Verification items for the finished model (mm, model axes). Face numbers are marked on the shaded views. A direction names the side the tool comes from. Coordinates: 2 decimals unless noted, no trailing zeros. Write each loop counter-clockwise with the first axis right and the second up, starting at its lowest first coordinate (ties: lowest second). Pieces come first, ordered by that corner, then holes. Notation, with made-up numbers: (-38, 47) -> (1, 47) arc R32 ccw to (1, 86) -> close; hole circle Ø3 at (-29.75, 52). An arc over 180 degrees is marked (long way). Answer in a Markdown table with one row per item.
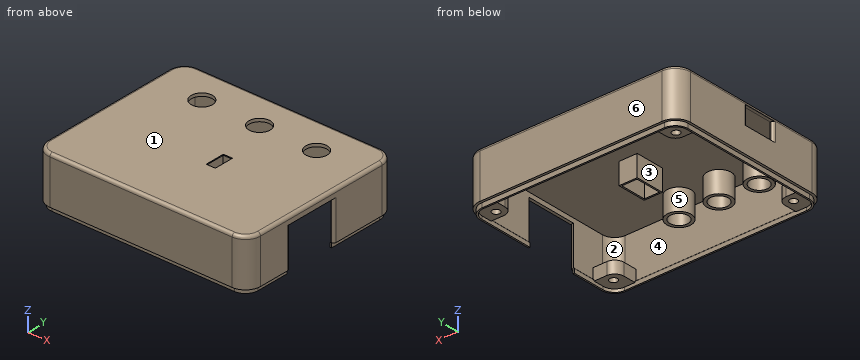
```python
from build123d import *

# Parameters (mm, degrees)
CYLINDER019_R     = 1.25
CYLINDER019_DEPTH = 10
CYLINDER018_R     = 1.25
CYLINDER018_DEPTH = 10
CYLINDER017_R     = 1.25
CYLINDER017_DEPTH = 10
BOX005_W          = 5
BOX005_H          = 8.5
BOX005_DEPTH      = 13.5
BOX006_W          = 3
BOX006_H          = 6.5
BOX006_DEPTH      = 14.5
CYLINDER015_R     = 3
CYLINDER015_DEPTH = 7.6
CYLINDER013_R     = 3
CYLINDER013_DEPTH = 7.6
CYLINDER011_R     = 3
CYLINDER011_DEPTH = 7.6
BOX003_W          = 10
BOX003_H          = 10
BOX003_DEPTH      = 6
CYLINDER002_R     = 3.5
CYLINDER002_DEPTH = 10
CYLINDER001_R     = 3.5
CYLINDER001_DEPTH = 10
CYLINDER_R        = 3.5
CYLINDER_DEPTH    = 10
BOX001_W          = 24
BOX001_H          = 16.8
BOX001_DEPTH      = 14.5
CYLINDER020_R     = 1.25
CYLINDER020_DEPTH = 10
BOX011_W          = 7.5
BOX011_H          = 7.5
BOX011_DEPTH      = 4
FILLET003_1_R     = 4
FILLET003_2_R     = 3
BOX010_W          = 7.5
BOX010_H          = 7.5
BOX010_DEPTH      = 4
FILLET002_1_R     = 4
FILLET002_2_R     = 3
BOX009_W          = 7.5
BOX009_H          = 7.5
BOX009_DEPTH      = 4
FILLET001_1_R     = 4
FILLET001_2_R     = 3
BOX004_W          = 6
BOX004_H          = 9.5
BOX004_DEPTH      = 7
CYLINDER012_R     = 4
CYLINDER012_DEPTH = 7
CYLINDER014_R     = 4
CYLINDER014_DEPTH = 7
CYLINDER016_R     = 4
CYLINDER016_DEPTH = 7
BOX008_W          = 7.5
BOX008_H          = 7.5
BOX008_DEPTH      = 4
FILLET_1_R        = 4
FILLET_2_R        = 3
BOX016_W          = 67.4
BOX016_H          = 53.4
BOX016_DEPTH      = 1.5
FILLET009_R       = 3.8
BOX013_W          = 68.4
BOX013_H          = 54.4
BOX013_DEPTH      = 1.5
FILLET008_R       = 4.2
BOX002_W          = 68
BOX002_H          = 54
BOX002_DEPTH      = 14.5
FILLET007_R       = 4
THICKNESS001_T    = 1
FILLET010_1_R     = 0.8
FILLET010_2_R     = 0.2


with BuildPart() as obj1:
    # Cylinder019 → Cylinder019 (new body)
    with BuildSketch(Plane(origin=(63.75, 49.15, -2), x_dir=(1, 0, 0), z_dir=(0, 0, 1))):
        Circle(CYLINDER019_R)
    extrude(amount=CYLINDER019_DEPTH)


with BuildPart() as obj2:
    # Cylinder018 → Cylinder018 (new body)
    with BuildSketch(Plane(origin=(4.5, 49.15, -2), x_dir=(1, 0, 0), z_dir=(0, 0, 1))):
        Circle(CYLINDER018_R)
    extrude(amount=CYLINDER018_DEPTH)


with BuildPart() as obj3:
    # Cylinder017 → Cylinder017 (new body)
    with BuildSketch(Plane(origin=(4.5, 4.65, -2), x_dir=(1, 0, 0), z_dir=(0, 0, 1))):
        Circle(CYLINDER017_R)
    extrude(amount=CYLINDER017_DEPTH)


with BuildPart() as obj4:
    # Box005 → Box005 (new body)
    with BuildSketch(Plane(origin=(35.75, 19.5, 6.2), x_dir=(1, 0, 0), z_dir=(0, 0, 1))):
        with Locations((2.5, 4.25)):
            Rectangle(BOX005_W, BOX005_H)
    extrude(amount=BOX005_DEPTH)


with BuildPart() as obj5:
    # Box006 → Box006 (new body)
    with BuildSketch(Plane(origin=(36.75, 20.5, 6.2), x_dir=(1, 0, 0), z_dir=(0, 0, 1))):
        with Locations((1.5, 3.25)):
            Rectangle(BOX006_W, BOX006_H)
    extrude(amount=BOX006_DEPTH)

    # Fusion: union obj4
    add(obj4.part)


with BuildPart() as ledhole002:
    # Cylinder015 → Cylinder015 (new body)
    with BuildSketch(Plane(origin=(40.9, 6.2, 12), x_dir=(1, 0, 0), z_dir=(0, 0, 1))):
        Circle(CYLINDER015_R)
    extrude(amount=CYLINDER015_DEPTH)


with BuildPart() as ledhole001:
    # Cylinder013 → Cylinder013 (new body)
    with BuildSketch(Plane(origin=(27.7, 6.2, 12), x_dir=(1, 0, 0), z_dir=(0, 0, 1))):
        Circle(CYLINDER013_R)
    extrude(amount=CYLINDER013_DEPTH)


with BuildPart() as ledhole:
    # Cylinder011 → Cylinder011 (new body)
    with BuildSketch(Plane(origin=(14.5, 6.2, 12), x_dir=(1, 0, 0), z_dir=(0, 0, 1))):
        Circle(CYLINDER011_R)
    extrude(amount=CYLINDER011_DEPTH)


with BuildPart() as usbhole:
    # Box003 → Box003 (new body)
    with BuildSketch(Plane(origin=(-3, 18.7, 12.8), x_dir=(1, 0, 0), z_dir=(0, 0, 1))):
        with Locations((5, 5)):
            Rectangle(BOX003_W, BOX003_H)
    extrude(amount=BOX003_DEPTH)


with BuildPart() as pothole002:
    # Cylinder002 → Cylinder002 (new body)
    with BuildSketch(Plane(origin=(53, 43.6, 11), x_dir=(1, 0, 0), z_dir=(0, 0, 1))):
        Circle(CYLINDER002_R)
    extrude(amount=CYLINDER002_DEPTH)


with BuildPart() as pothole001:
    # Cylinder001 → Cylinder001 (new body)
    with BuildSketch(Plane(origin=(34.25, 43.6, 11), x_dir=(1, 0, 0), z_dir=(0, 0, 1))):
        Circle(CYLINDER001_R)
    extrude(amount=CYLINDER001_DEPTH)


with BuildPart() as pothole:
    # Cylinder → Cylinder (new body)
    with BuildSketch(Plane(origin=(15.25, 43.6, 11), x_dir=(1, 0, 0), z_dir=(0, 0, 1))):
        Circle(CYLINDER_R)
    extrude(amount=CYLINDER_DEPTH)


with BuildPart() as obj6:
    # Box001 → Box001 (new body)
    with BuildSketch(Plane(origin=(47, 15, 3), x_dir=(1, 0, 0), z_dir=(0, 0, 1))):
        with Locations((12, 8.4)):
            Rectangle(BOX001_W, BOX001_H)
    extrude(amount=BOX001_DEPTH)


with BuildPart() as topholes:
    # Cylinder020 → Cylinder020 (new body)
    with BuildSketch(Plane(origin=(63.75, 4.65, -2), x_dir=(1, 0, 0), z_dir=(0, 0, 1))):
        Circle(CYLINDER020_R)
    extrude(amount=CYLINDER020_DEPTH)

    # Fusion009: union obj1, obj2, obj3, obj5, ledhole002, ledhole001, ledhole, UsbHole, PotHole002, PotHole001, PotHole, obj6
    add(obj1.part)
    add(obj2.part)
    add(obj3.part)
    add(obj5.part)
    add(ledhole002.part)
    add(ledhole001.part)
    add(ledhole.part)
    add(usbhole.part)
    add(pothole002.part)
    add(pothole001.part)
    add(pothole.part)
    add(obj6.part)


with BuildPart() as obj7:
    # Box011 → Box011 (new body)
    with BuildSketch(Plane.XY.offset(4)):
        with Locations((3.75, 3.75)):
            Rectangle(BOX011_W, BOX011_H)
    extrude(amount=BOX011_DEPTH)

    # Fillet003 1
    fillet003_1_edges = [obj7.edges().sort_by_distance(p)[0] for p in [
        (7.5, 7.5, 6),
    ]]
    fillet(fillet003_1_edges, radius=FILLET003_1_R)

    # Fillet003 2
    fillet003_2_edges = [obj7.edges().sort_by_distance(p)[0] for p in [
        (0, 0, 6),
    ]]
    fillet(fillet003_2_edges, radius=FILLET003_2_R)


with BuildPart() as obj7_1:
    # Fillet003 placement: moved
    add(obj7.part.moved(Location((60.5, 46.5, 0))))


with BuildPart() as obj8:
    # Box010 → Box010 (new body)
    with BuildSketch(Plane.XY.offset(4)):
        with Locations((3.75, 3.75)):
            Rectangle(BOX010_W, BOX010_H)
    extrude(amount=BOX010_DEPTH)

    # Fillet002 1
    fillet002_1_edges = [obj8.edges().sort_by_distance(p)[0] for p in [
        (7.5, 0, 6),
    ]]
    fillet(fillet002_1_edges, radius=FILLET002_1_R)

    # Fillet002 2
    fillet002_2_edges = [obj8.edges().sort_by_distance(p)[0] for p in [
        (0, 7.5, 6),
    ]]
    fillet(fillet002_2_edges, radius=FILLET002_2_R)


with BuildPart() as obj8_1:
    # Fillet002 placement: moved
    add(obj8.part.moved(Location((60.5, 0, 0))))


with BuildPart() as obj9:
    # Box009 → Box009 (new body)
    with BuildSketch(Plane.XY.offset(4)):
        with Locations((3.75, 3.75)):
            Rectangle(BOX009_W, BOX009_H)
    extrude(amount=BOX009_DEPTH)

    # Fillet001 1
    fillet001_1_edges = [obj9.edges().sort_by_distance(p)[0] for p in [
        (0, 7.5, 6),
    ]]
    fillet(fillet001_1_edges, radius=FILLET001_1_R)

    # Fillet001 2
    fillet001_2_edges = [obj9.edges().sort_by_distance(p)[0] for p in [
        (7.5, 0, 6),
    ]]
    fillet(fillet001_2_edges, radius=FILLET001_2_R)


with BuildPart() as obj9_1:
    # Fillet001 placement: moved
    add(obj9.part.moved(Location((0, 46.5, 0))))


with BuildPart() as obj10:
    # Box004 → Box004 (new body)
    with BuildSketch(Plane(origin=(35.25, 19, 12), x_dir=(1, 0, 0), z_dir=(0, 0, 1))):
        with Locations((3, 4.75)):
            Rectangle(BOX004_W, BOX004_H)
    extrude(amount=BOX004_DEPTH)


with BuildPart() as ledtube:
    # Cylinder012 → Cylinder012 (new body)
    with BuildSketch(Plane(origin=(14.5, 6.2, 12), x_dir=(1, 0, 0), z_dir=(0, 0, 1))):
        Circle(CYLINDER012_R)
    extrude(amount=CYLINDER012_DEPTH)


with BuildPart() as ledtube001:
    # Cylinder014 → Cylinder014 (new body)
    with BuildSketch(Plane(origin=(27.7, 6.2, 12), x_dir=(1, 0, 0), z_dir=(0, 0, 1))):
        Circle(CYLINDER014_R)
    extrude(amount=CYLINDER014_DEPTH)


with BuildPart() as ledtube002:
    # Cylinder016 → Cylinder016 (new body)
    with BuildSketch(Plane(origin=(40.9, 6.2, 12), x_dir=(1, 0, 0), z_dir=(0, 0, 1))):
        Circle(CYLINDER016_R)
    extrude(amount=CYLINDER016_DEPTH)


with BuildPart() as obj11:
    # Box008 → Box008 (new body)
    with BuildSketch(Plane.XY.offset(4)):
        with Locations((3.75, 3.75)):
            Rectangle(BOX008_W, BOX008_H)
    extrude(amount=BOX008_DEPTH)

    # Fillet 1
    fillet_1_edges = [obj11.edges().sort_by_distance(p)[0] for p in [
        (0, 0, 6),
    ]]
    fillet(fillet_1_edges, radius=FILLET_1_R)

    # Fillet 2
    fillet_2_edges = [obj11.edges().sort_by_distance(p)[0] for p in [
        (7.5, 7.5, 6),
    ]]
    fillet(fillet_2_edges, radius=FILLET_2_R)


with BuildPart() as fillet009:
    # Box016 → Box016 (new body)
    with BuildSketch(Plane(origin=(0.3, 0.3, 3), x_dir=(1, 0, 0), z_dir=(0, 0, 1))):
        with Locations((33.7, 26.7)):
            Rectangle(BOX016_W, BOX016_H)
    extrude(amount=BOX016_DEPTH)

    # Fillet009
    fillet009_edges = [fillet009.edges().sort_by_distance(p)[0] for p in [
        (0.3, 0.3, 3.75),
        (0.3, 53.7, 3.75),
        (67.7, 0.3, 3.75),
        (67.7, 53.7, 3.75),
    ]]
    fillet(fillet009_edges, radius=FILLET009_R)


with BuildPart() as snaptop:
    # Box013 → Box013 (new body)
    with BuildSketch(Plane(origin=(-0.2, -0.2, 3), x_dir=(1, 0, 0), z_dir=(0, 0, 1))):
        with Locations((34.2, 27.2)):
            Rectangle(BOX013_W, BOX013_H)
    extrude(amount=BOX013_DEPTH)

    # Fillet008
    fillet008_edges = [snaptop.edges().sort_by_distance(p)[0] for p in [
        (-0.2, -0.2, 3.75),
        (-0.2, 54.2, 3.75),
        (68.2, -0.2, 3.75),
        (68.2, 54.2, 3.75),
    ]]
    fillet(fillet008_edges, radius=FILLET008_R)

    # Cut: cut Fillet009
    add(fillet009.part, mode=Mode.SUBTRACT)


with BuildPart() as top:
    # Box002 → Box002 (new body)
    with BuildSketch(Plane.XY.offset(4.5)):
        with Locations((34, 27)):
            Rectangle(BOX002_W, BOX002_H)
    extrude(amount=BOX002_DEPTH)

    # Fillet007
    fillet007_edges = [top.edges().sort_by_distance(p)[0] for p in [
        (0, 0, 11.75),
        (0, 54, 11.75),
        (68, 0, 11.75),
        (68, 54, 11.75),
    ]]
    fillet(fillet007_edges, radius=FILLET007_R)

    # Thickness001
    thickness001_openings = [top.faces().sort_by_distance(p)[0] for p in [
        (34, 27, 4.5),
    ]]
    offset(amount=THICKNESS001_T, openings=thickness001_openings)

    # Fusion008: union obj7, obj8, obj9, PotHole, obj10, ledtube, ledtube001, ledtube002, obj11, snaptop
    add(obj7_1.part)
    add(obj8_1.part)
    add(obj9_1.part)
    add(pothole.part)
    add(obj10.part)
    add(ledtube.part)
    add(ledtube001.part)
    add(ledtube002.part)
    add(obj11.part)
    add(snaptop.part)

    # Cut004: cut TopHoles
    add(topholes.part, mode=Mode.SUBTRACT)

    # Fillet010 1
    fillet010_1_edges = [top.edges().sort_by_distance(p)[0] for p in [
        (-1, 28.7, 15.8),
        (-1, 18.7, 15.8),
        (69, 31.8, 11),
        (69, 15, 11),
    ]]
    fillet(fillet010_1_edges, radius=FILLET010_1_R)

    # Fillet010 2
    fillet010_2_edges = [top.edges().sort_by_distance(p)[0] for p in [
        (0.3, 27, 4.5),
        (34, 0.3, 4.5),
        (34, 53.7, 4.5),
        (67.7, 39.15, 4.5),
        (67.7, 11.25, 4.5),
    ]]
    fillet(fillet010_2_edges, radius=FILLET010_2_R)


solid = top.part
```
1. Access from +Z, -Z, +X, -X, +Y, -Y to the whole of each face (thin tool, end or side, straight path). Record for the marked faces 4, 5 and 6.
Findings below:
| item | result |
|---|---|
| face 4 | none |
| face 5 | -Z |
| face 6 | +Z, -Z, +X, -X, +Y |
2. Material ranges on probe 1 along Y at (x, z) = (63.75, 6.95); probe 2 along X at (y, z) = (4.65, 7.15); probe 3 along Y at (x, z) = (6, 16.5), recorded low to high. Write a range as from..to.
Findings below:
| item | result |
|---|---|
| probe 1 | y = -1..3.4, 5.9..7.5, 46.5..47.9, 50.4..55 |
| probe 2 | x = -1..3.25, 5.75..7.5, 60.5..62.5, 65..69 |
| probe 3 | y = -1..0, 54..55 |
3. Go/stop test with flat-tipped pins: pin 1 (1.6 mm diameter, centred on y = 37.5, z = 4, fed in from -X); pin 2 (1.4 mm diameter, centred on y = 19.5, z = 4, fed in from +X); pin 3 (1 mm diameter, centred on x = 24, y = 33, fed in from -Z); pin 4 (0.6 mm diameter, centred on x = 45, z = 3.5, fed in from +Y). Record where each tip stops, or that it passes through.
Findings below:
| item | result |
|---|---|
| pin 1 | stops at x = -1 |
| pin 2 | stops at x = 0.3 |
| pin 3 | stops at z = 19 |
| pin 4 | stops at y = 54.2 |
4. Sectioned sample at A-A, the plane x = 53. Record the cut outline in (y, z).
Findings below:
| item | result |
|---|---|
| outline | (-1, 4.5) -> (-0.2, 4.5) -> (-0.2, 3) -> (0.3, 3) -> (0.3, 4.3) arc R0.2 ccw to (0.1, 4.5) -> (0, 4.5) -> (0, 19) -> (40.1, 19) -> (40.1, 20) -> (0, 20) arc R1 ccw to (-1, 19) -> close; (47.1, 19) -> (54, 19) -> (54, 4.5) -> (53.9, 4.5) arc R0.2 ccw to (53.7, 4.3) -> (53.7, 3) -> (54.2, 3) -> (54.2, 4.5) -> (55, 4.5) -> (55, 19) arc R1 ccw to (54, 20) -> (47.1, 20) -> close |
5. Sectioned sample at D-D, the plane y = 13. Record the cut outline in (x, z), and give its area (3 significant figures).
Findings below:
| item | result |
|---|---|
| outline | (-1, 4.5) -> (-0.2, 4.5) -> (-0.2, 3) -> (0.3, 3) -> (0.3, 4.3) arc R0.2 ccw to (0.1, 4.5) -> (0, 4.5) -> (0, 19) -> (68, 19) -> (68, 4.5) -> (67.9, 4.5) arc R0.2 ccw to (67.7, 4.3) -> (67.7, 3) -> (68.2, 3) -> (68.2, 4.5) -> (69, 4.5) -> (69, 19) arc R1 ccw to (68, 20) -> (0, 20) arc R1 ccw to (-1, 19) -> close |
| area | 100 mm² |
6. Release check for a two-part mould opening along Z. For the marked faces 1, 2 and 3 record: released by +Z, released by -Z, zero draft, split by the parting line, or undercut.
Findings below:
| item | result |
|---|---|
| face 1 | released by +Z |
| face 2 | undercut |
| face 3 | zero draft |
7. Sectioned sample at B-B, the plane z = 6.75. Count the separate pieces of the cut face and the enclosed holes in it, and give its area (3 significant figures).
Findings below:
| item | result |
|---|---|
| separate pieces | 1 |
| enclosed holes | 4 |
| area | 407 mm² |
